```python
from build123d import *

# Parameters (mm, degrees)
SKETCH1_R               = 161.4
SKETCH1_R_2             = 136
BOSS_EXTRUDE1_DEPTH     = 6.35
F_1_4_CLEARANCE_HOLE1_D = 6.7564
CIRPATTERN1_COUNT       = 4


with BuildPart() as part:
    # Sketch1 → Boss-Extrude1 (new body)
    with BuildSketch(Plane(origin=(0, 0, 0), x_dir=(1, 0, 0), z_dir=(0, 1, 0))):
        with Locations(Location((0, 0, 0), (0, 0, 270))):
            Circle(SKETCH1_R)
        with Locations(Location((0, 0, 0), (0, 0, 270))):
            Circle(SKETCH1_R_2, mode=Mode.SUBTRACT)
    extrude(amount=BOSS_EXTRUDE1_DEPTH)

    # 1/4 Clearance Hole1 (through all)
    with Locations(Plane(origin=(0, 6.35, 0), x_dir=(1, 0, 0), z_dir=(0, 1, 0))):
        with Locations((0, -148.7)):
            f_1_4_clearance_hole1 = Hole(F_1_4_CLEARANCE_HOLE1_D / 2)

    # CirPattern1: 1/4 Clearance Hole1 ×4 about axis
    cirpattern1_axis = Axis((0, 0, 0), (0, 1, 0))
    for i in range(1, CIRPATTERN1_COUNT):
        add(f_1_4_clearance_hole1.rotate(cirpattern1_axis, i * 360 / CIRPATTERN1_COUNT), mode=Mode.SUBTRACT)


solid = part.part
```
The model under review builds one solid part; all positions refer to its coordinate system, in mm. Give positions to 0.01 mm unless a question says otherwise; leave off trailing zeros. Write each loop counter-clockwise with the first axis right and the second up, starting at its lowest first coordinate (ties: lowest second). Pieces come first, ordered by that corner, then holes. Notation, with made-up numbers: (-17.5, -29.75) -> (34.5, -29.75) arc R12 cw to (34.5, -10.75) -> close; hole circle Ø1 at (39.5, 32.5). An arc over 180 degrees is marked (long way). Put each result on its own line as item: value.
(1) For pin 1 Ø1.5 at (y, z) = (2, 100.5) entering from +X; pin 2 Ø2 at (x, y) = (-57, 1.5) entering from -Z; pin 3 Ø1 at (x, y) = (16.5, 2.5) entering from -Z (3 decimals), all flat-tipped, find the tip position at first contact; note any pin that passes through.
Results are:
pin 1: x = 126.89
pin 2: z = -151.37
pin 3: z = -160.605
(2) We need section A-A, the plane z = 15.5. Give the boundary of the cut face in (x, y).
Results are:
outline: (-160.65, 0) -> (-135.11, 0) -> (-135.11, 6.35) -> (-160.65, 6.35) -> close; (135.11, 0) -> (160.65, 0) -> (160.65, 6.35) -> (135.11, 6.35) -> close
(3) We need section C-C, the plane x = 119. Give the boundary of the cut face in (y, z), and give its area (3 significant figures).
Results are:
outline: (0, -109.04) -> (6.35, -109.04) -> (6.35, -65.84) -> (0, -65.84) -> close; (0, 65.84) -> (6.35, 65.84) -> (6.35, 109.04) -> (0, 109.04) -> close
area: 549 mm²
(4) To check wall thickness, follow probe 1 along X at (y, z) = (4.25, 0); probe 2 along Z at (x, y) = (58, 6); probe 3 along Z at (x, y) = (-148.7, 2.5). State the ranges of each line that lie inside material, in increasing order. Write a range as from..to.
Results are:
probe 1: -161.4..-152.08, -145.32..-136, 136..145.32, 152.08..161.4
probe 2: -150.62..-123.01, 123.01..150.62
probe 3: -62.76..-3.38, 3.38..62.76
(5) We need section B-B, the plane y = 4. Give the boundary of the cut face in (x, z).
Results are:
outline: circle Ø322.8 at (0, 0); hole circle Ø6.76 at (-148.7, 0); hole circle Ø272 at (0, 0); hole circle Ø6.76 at (0, -148.7); hole circle Ø6.76 at (0, 148.7); hole circle Ø6.76 at (148.7, 0)
